from build123d import *

# Parameters (mm, degrees)
EXTRUDE_1_DEPTH     = 1.6
SKETCH_3_R          = 1.5
CUT_EXTRUDE_1_DEPTH = 1.6
SKETCH_8_W          = 8
SKETCH_8_H          = 15.5
EXTRUDE_2_DEPTH     = 16
SHELL_1_T           = -0.6
SKETCH_11_R         = 1.5
EXTRUDE_3_DEPTH     = 14
SKETCH_12_W         = 38
SKETCH_12_H         = 5
EXTRUDE_4_DEPTH     = 8
SKETCH_17_W         = 38.038888129
SKETCH_17_H         = 5
SKETCH_17_W_2       = 38
EXTRUDE_5_DEPTH     = 1


with BuildPart() as part:
    # 草图2 → 凸台-拉伸1 (new body)
    with BuildSketch(Plane(origin=(0, 0, 0), x_dir=(1, 0, 0), z_dir=(0, 1, 0))):
        with BuildLine():
            Line((-82.363056433, 39.03274813), (-15.363056433, 39.03274813))
            ThreePointArc((-15.363056433, 39.03274813), (-14.302396261, 38.593408302), (-13.863056433, 37.53274813))
            Line((-13.863056433, 37.53274813), (-13.863056433, 15.53274813))
            ThreePointArc((-13.863056433, 15.53274813), (-14.302396261, 14.472087958), (-15.363056433, 14.03274813))
            Line((-15.363056433, 14.03274813), (-82.363056433, 14.03274813))
            ThreePointArc((-82.363056433, 14.03274813), (-83.423716605, 14.472087958), (-83.863056433, 15.53274813))
            Line((-83.863056433, 15.53274813), (-83.863056433, 37.53274813))
            ThreePointArc((-83.863056433, 37.53274813), (-83.423716605, 38.593408302), (-82.363056433, 39.03274813))
        make_face()
    extrude(amount=EXTRUDE_1_DEPTH)

    # 草图3 → 切除-拉伸1 (cut)
    with BuildSketch(Plane(origin=(0, 1.6, 0), x_dir=(1, 0, 0), z_dir=(0, 1, 0))):
        with Locations(Location((-80.863056433, 36.03274813, 0), (0, 0, 270))):
            Circle(SKETCH_3_R)
        with Locations(Location((-16.863056433, 36.03274813, 0), (0, 0, 270))):
            Circle(SKETCH_3_R)
        with Locations(Location((-16.863056433, 17.03274813, 0), (0, 0, 90))):
            Circle(SKETCH_3_R)
        with Locations(Location((-80.863056433, 17.03274813, 0), (0, 0, 90))):
            Circle(SKETCH_3_R)
    extrude(amount=-CUT_EXTRUDE_1_DEPTH, mode=Mode.SUBTRACT)

    # 草图8 → 凸台-拉伸2 (add)
    with BuildSketch(Plane(origin=(0, 1.6, 0), x_dir=(1, 0, 0), z_dir=(0, 1, 0))):
        with Locations((-72.863056433, 26.78274813)):
            Rectangle(SKETCH_8_W, SKETCH_8_H)
        with Locations((-24.863056433, 26.28274813)):
            Rectangle(SKETCH_8_W, SKETCH_8_H)
    extrude(amount=EXTRUDE_2_DEPTH)

    # 抽壳1
    shell_1_openings = [part.faces().sort_by_distance(p)[0] for p in [
        (-72.863056433, 17.6, -26.78274813),
        (-24.863056433, 17.6, -26.28274813),
    ]]
    offset(amount=SHELL_1_T, openings=shell_1_openings, kind=Kind.INTERSECTION)

    # 草图11 → 凸台-拉伸3 (add)
    with BuildSketch(Plane(origin=(0, 0.6, 0), x_dir=(1, 0, 0), z_dir=(0, 1, 0))):
        with Locations(Location((-72.863056433, 30.03274813, 0), (0, 0, 270))):
            Circle(SKETCH_11_R)
        with Locations(Location((-72.863056433, 23.53274813, 0), (0, 0, 270))):
            Circle(SKETCH_11_R)
        with Locations(Location((-24.863056433, 30.03274813, 0), (0, 0, 270))):
            Circle(SKETCH_11_R)
        with Locations(Location((-24.863056433, 23.53274813, 0), (0, 0, 270))):
            Circle(SKETCH_11_R)
    extrude(amount=EXTRUDE_3_DEPTH)

    # 草图12 → 凸台-拉伸4 (add)
    with BuildSketch(Plane(origin=(0, 1.6, 0), x_dir=(1, 0, 0), z_dir=(0, 1, 0))):
        with Locations((-48.863056433, 32.03274813)):
            Rectangle(SKETCH_12_W, SKETCH_12_H)
        with Locations((-48.863056433, 21.03274813)):
            Rectangle(SKETCH_12_W, SKETCH_12_H)
    extrude(amount=EXTRUDE_4_DEPTH)

    # 草图17 → 凸台-拉伸5 (add)
    with BuildSketch(Plane.XZ):
        with Locations((-48.843612369, -21.03274813)):
            Rectangle(SKETCH_17_W, SKETCH_17_H)
        with Locations((-48.863056433, -32.03274813)):
            Rectangle(SKETCH_17_W_2, SKETCH_17_H)
    extrude(amount=EXTRUDE_5_DEPTH)


solid = part.part
Work out the finished part from the listing and answer in its coordinate system (mm). A direction names the side the tool comes from. Give positions to 0.01 mm unless a question says otherwise; leave off trailing zeros. Loops run counter-clockwise (first coordinate to the right, second up) from the corner with the lowest first, then second, coordinate; pieces in that order, holes last. Notation, with made-up numbers: (-1, -13.5) - (44, -13.5) arc R26 cw to (44, 24.5) - close; hole circle Ø1 at (-21, 9). An arc over 180 degrees is marked (long way). Answer in a Markdown table with one row per item.
(1) Section A-A (y = 16) is taken. Give the vertices of the cut face in (x, z).
Results list:
| item | result |
|---|---|
| outline | (-76.86, -34.53) - (-68.86, -34.53) - (-68.86, -19.03) - (-76.86, -19.03) - close; (-28.86, -34.03) - (-20.86, -34.03) - (-20.86, -18.53) - (-28.86, -18.53) - close; hole (-76.26, -33.93) - (-69.46, -33.93) - (-69.46, -19.63) - (-76.26, -19.63) - close; hole (-28.26, -33.43) - (-21.46, -33.43) - (-21.46, -19.13) - (-28.26, -19.13) - close |
(2) Section B-B (z = -25.75) is taken. Give the vertices of the cut face in (x, y), and give its area (3 significant figures).
Results list:
| item | result |
|---|---|
| outline | (-83.86, 0) - (-13.86, 0) - (-13.86, 1.6) - (-20.86, 1.6) - (-20.86, 17.6) - (-21.46, 17.6) - (-21.46, 1) - (-14.46, 1) - (-14.46, 0.6) - (-83.26, 0.6) - (-83.26, 1) - (-76.26, 1) - (-76.26, 17.6) - (-76.86, 17.6) - (-76.86, 1.6) - (-83.86, 1.6) - close; (-69.46, 1) - (-28.26, 1) - (-28.26, 17.6) - (-28.86, 17.6) - (-28.86, 1.6) - (-68.86, 1.6) - (-68.86, 17.6) - (-69.46, 17.6) - close |
| area | 115 mm² |
(3) Flat-ended cylindrical pins translate along their axes: pin 1 Ø7 at (y, z) = (8, -26) entering from +X; pin 2 Ø4.5 at (y, z) = (9, -24.5) entering from -X; pin 3 Ø0.5 at (y, z) = (-0.5, -33) entering from -X. Find the tip coordinate at first contact, or state that the pin passes through.
Results list:
| item | result |
|---|---|
| pin 1 | stops at x = -20.86 |
| pin 2 | stops at x = -76.86 |
| pin 3 | stops at x = -67.86 |
(4) Section D-D (x = -52) is taken. Give the vertices of the cut face in (y, z).
Results list:
| item | result |
|---|---|
| outline | (-1, -34.53) - (0, -34.53) - (0, -39.03) - (1.6, -39.03) - (1.6, -34.53) - (9.6, -34.53) - (9.6, -29.53) - (1.6, -29.53) - (1.6, -23.53) - (9.6, -23.53) - (9.6, -18.53) - (1.6, -18.53) - (1.6, -14.03) - (0, -14.03) - (0, -18.53) - (-1, -18.53) - (-1, -23.53) - (0, -23.53) - (0, -29.53) - (-1, -29.53) - close; hole (0.6, -38.43) - (1, -38.43) - (1, -14.63) - (0.6, -14.63) - close |
(5) A tool of negligible diameter and unlimited length cuts with its end or side. For faces 1 (the face through (-73, 14.6, -24)), 2 (the face through (-68.863, 9, -27)), 3 (the face through (-48, 1, -27)), from which of +Z, -Z, +X, -X, +Y, -Y can it reach the whole face along a straight path? Write none if from no direction.
Results list:
| item | result |
|---|---|
| face 1 | +Y |
| face 2 | +Z, -Z, +Y |
| face 3 | none |
(6) Consider L1, parallel to X at y = 12.75, z = -22; L2, parallel to X at y = 1.5, z = -26; L3, parallel to X at y = 4, z = -21.75. Determine where each line is inside the solid, lowest interval first. Write a range as [from, to].
Results list:
| item | result |
|---|---|
| L1 | x = [-76.86, -76.26], [-69.46, -68.86], [-28.86, -28.26], [-21.46, -20.86] |
| L2 | x = [-83.86, -76.26], [-69.46, -28.26], [-21.46, -13.86] |
| L3 | x = [-76.86, -76.26], [-69.46, -68.86], [-67.86, -29.86], [-28.86, -28.26], [-21.46, -20.86] |
(7) Section C-C (y = 2.75) is taken. State how many separate pieces and enclosed holes the cut face has, and give its area (3 significant figures).
Results list:
| item | result |
|---|---|
| separate pieces | 8 |
| enclosed holes | 2 |
| area | 462 mm² |
(8) For a pull along Z with two mould halves and no side action, classify faces 4 (the face through (-76.263, 9, -27)), 5 (the face through (-73, 9, -19.033)), 6 (the face through (-25, 9, -19.133)), 7 (the face through (-67.863, 6, -21)) as pulls with the +Z half, pulls with the -Z half, needs draft (parallel to the pull), parting line crosses it, or undercut.
Results list:
| item | result |
|---|---|
| face 4 | undercut |
| face 5 | pulls with the +Z half |
| face 6 | undercut |
| face 7 | needs draft |
